```python
from build123d import *

# Parameters (mm, degrees)
SKETCH_1_W          = 42
SKETCH_1_H          = 23.5
SKETCH_1_R          = 1.25
SKETCH_1_R_2        = 1.2
EXTRUDE_1_DEPTH     = 3
FILLET_1_R          = 4
SKETCH_2_R          = 2.6
CUT_EXTRUDE_1_DEPTH = 1.5


with BuildPart() as part:
    # 草图1 → 凸台-拉伸1 (new body)
    with BuildSketch(Plane(origin=(0, 0, 0), x_dir=(1, 0, 0), z_dir=(0, 1, 0))):
        Rectangle(SKETCH_1_W, SKETCH_1_H)
        with Locations(Location((7, 0, 0), (0, 0, 270))):
            Circle(SKETCH_1_R, mode=Mode.SUBTRACT)
        with Locations(Location((0, -7, 0), (0, 0, 270))):
            Circle(SKETCH_1_R, mode=Mode.SUBTRACT)
        with Locations(Location((-7, 0, 0), (0, 0, 270))):
            Circle(SKETCH_1_R, mode=Mode.SUBTRACT)
        with Locations(Location((0, 7, 0), (0, 0, 270))):
            Circle(SKETCH_1_R, mode=Mode.SUBTRACT)
        with Locations(Location((-17.9, 8.65, 0), (0, 0, 270))):
            Circle(SKETCH_1_R_2, mode=Mode.SUBTRACT)
        with Locations(Location((17.9, 8.65, 0), (0, 0, 90))):
            Circle(SKETCH_1_R_2, mode=Mode.SUBTRACT)
        with Locations(Location((-17.9, -8.65, 0), (0, 0, 90))):
            Circle(SKETCH_1_R_2, mode=Mode.SUBTRACT)
        with Locations(Location((17.9, -8.65, 0), (0, 0, 270))):
            Circle(SKETCH_1_R_2, mode=Mode.SUBTRACT)
    extrude(amount=EXTRUDE_1_DEPTH)

    # 圆角1
    fillet_1_edges = [part.edges().sort_by_distance(p)[0] for p in [
        (-21, 1.5, -11.75),
        (21, 1.5, -11.75),
        (21, 1.5, 11.75),
        (-21, 1.5, 11.75),
    ]]
    fillet(fillet_1_edges, radius=FILLET_1_R)

    # 草图2 → 切除-拉伸1 (cut)
    with BuildSketch(Plane(origin=(0, 3, 0), x_dir=(1, 0, 0), z_dir=(0, 1, 0))):
        with Locations(Location((7, 0, 0), (0, 0, 270))):
            Circle(SKETCH_2_R)
        with Locations(Location((0, -7, 0), (0, 0, 270))):
            Circle(SKETCH_2_R)
        with Locations(Location((-7, 0, 0), (0, 0, 270))):
            Circle(SKETCH_2_R)
        with Locations(Location((0, 7, 0), (0, 0, 270))):
            Circle(SKETCH_2_R)
    extrude(amount=-CUT_EXTRUDE_1_DEPTH, mode=Mode.SUBTRACT)


solid = part.part
```
CAD build for the part. Positions are in the model's coordinates, mm. A direction names the side the tool comes from. Round coordinates to 2 decimals unless told otherwise and drop trailing zeros. Order: outer loops, then holes, each group sorted by start corner. A loop starts at its lowest first (then second) coordinate and runs counter-clockwise, first axis right, second up.
Q1. Which spindle directions (+Z, -Z, +X, -X, +Y, -Y) get a long thin tool onto all of the face, cutting with end or side? Do faces 4 (the flat face through (21, 1, 0)), 5 (the cylindrical face through (0.78, 2.26, -4.52)). Say none if no direction does.
Q2. Wall check: L1, parallel to Z at x = 0, y = 1; L2, parallel to X at y = 2.3, z = 0; L3, parallel to Z at x = 7, y = 0.4. Give the ranges that are in metal, low to high.
Q3. Slice it at A-A (x = 7). Write the cut outline in (y, z), and give its area (4 significant figures).
Q4. Slice it at B-B (y = 1.1). State how many separate pieces and enclosed holes the cut face has, and give its area (3 significant figures).
Q5. Slice it at C-C (z = 0). Write the cut outline in (x, y), and give its area (3 significant figures).
Q6. Slice it at D-D (z = -7). Write the cut outline in (x, y).
Q7. Drop a flat-ended pin along its axis: pin 1 (1.6 mm diameter, centred on x = -7.5, z = -1, fed in from +Y). Give the stop position or say it passes through.
Q8. Two-plate mould, pull along X, no slides. Class faces 1 (the cylindrical face through (19.797, 1.521, -10.609)), 2 (the flat face through (-21, 1, 0)), 3 (the flat face through (8, 1.5, 1)): pulls with the +X half, pulls with the -X half, needs draft (parallel to the pull), parting line crosses it, or undercut.
Results below:
1. face 4: +Z, -Z, +X, +Y, -Y
1. face 5: +Y
2. L1: z = -11.75 to -8.25, -5.75 to 5.75, 8.25 to 11.75
2. L2: x = -21 to -9.6, -4.4 to 4.4, 9.6 to 21
2. L3: z = -11.75 to -1.25, 1.25 to 11.75
3. outline: (0, -11.75) - (3, -11.75) - (3, -2.6) - (1.5, -2.6) - (1.5, -1.25) - (0, -1.25) - close; (0, 1.25) - (1.5, 1.25) - (1.5, 2.6) - (3, 2.6) - (3, 11.75) - (0, 11.75) - close
3. area: 58.95 mm2
4. separate pieces: 1
4. enclosed holes: 8
4. area: 936 mm2
5. outline: (-21, 0) - (-8.25, 0) - (-8.25, 1.5) - (-9.6, 1.5) - (-9.6, 3) - (-21, 3) - close; (-5.75, 0) - (5.75, 0) - (5.75, 1.5) - (4.4, 1.5) - (4.4, 3) - (-4.4, 3) - (-4.4, 1.5) - (-5.75, 1.5) - close; (8.25, 0) - (21, 0) - (21, 3) - (9.6, 3) - (9.6, 1.5) - (8.25, 1.5) - close
5. area: 103 mm2
6. outline: (-21, 0) - (-1.25, 0) - (-1.25, 1.5) - (-2.6, 1.5) - (-2.6, 3) - (-21, 3) - close; (1.25, 0) - (21, 0) - (21, 3) - (2.6, 3) - (2.6, 1.5) - (1.25, 1.5) - close
7. pin 1: stops at y = 1.5
8. face 1: pulls with the +X half
8. face 2: pulls with the -X half
8. face 3: undercut
